Answer from the drawing. Dimensions are ordinates in mm from the lowest x, y and z of the part. Round coordinates to 2 decimals unless told otherwise and drop trailing zeros. Order: outer loops, then holes, each group sorted by start corner. A loop starts at its lowest first (then second) coordinate and runs counter-clockwise, first axis right, second up. Notation, with made-up numbers: (79, 67.25) -> (121, 67.25) arc R14 cw to (121, 74.25) -> close; hole circle Ø5 at (20.25, -2.5). An arc over 180 degrees is marked (long way). Use a Markdown table: item, result. Add a question column.
Item 1: Find the intervals of material crossed by L1, parallel to Z at x = 80, y = 63.5; L2, parallel to Z at x = 46, y = 53, in increasing order. Write a range as [from, to].
Item 2: A flat-ended cylindrical pin translates along its axis: P1, Ø4, axis at x = 98.5, y = 78.5, coming from the -Z side. Find the tip coordinate at first contact, or state that the pin passes through.
Item 3: For a pull along Z with two mould halves and no side action, classify the marked faces 1, 2, 3 and 4 as +Z half, -Z half, draft (parallel to the pull), parting line (faces both ways), or undercut.
Item 4: A cutting plane is placed at A-A, the plane y = 63.5. Determine the outline of the cut face in (x, z), plus the area to 3 significant figures.
Item 5: A cutting plane is placed at C-C, the plane x = 63.5. Determine the outline of the cut face in (y, z).
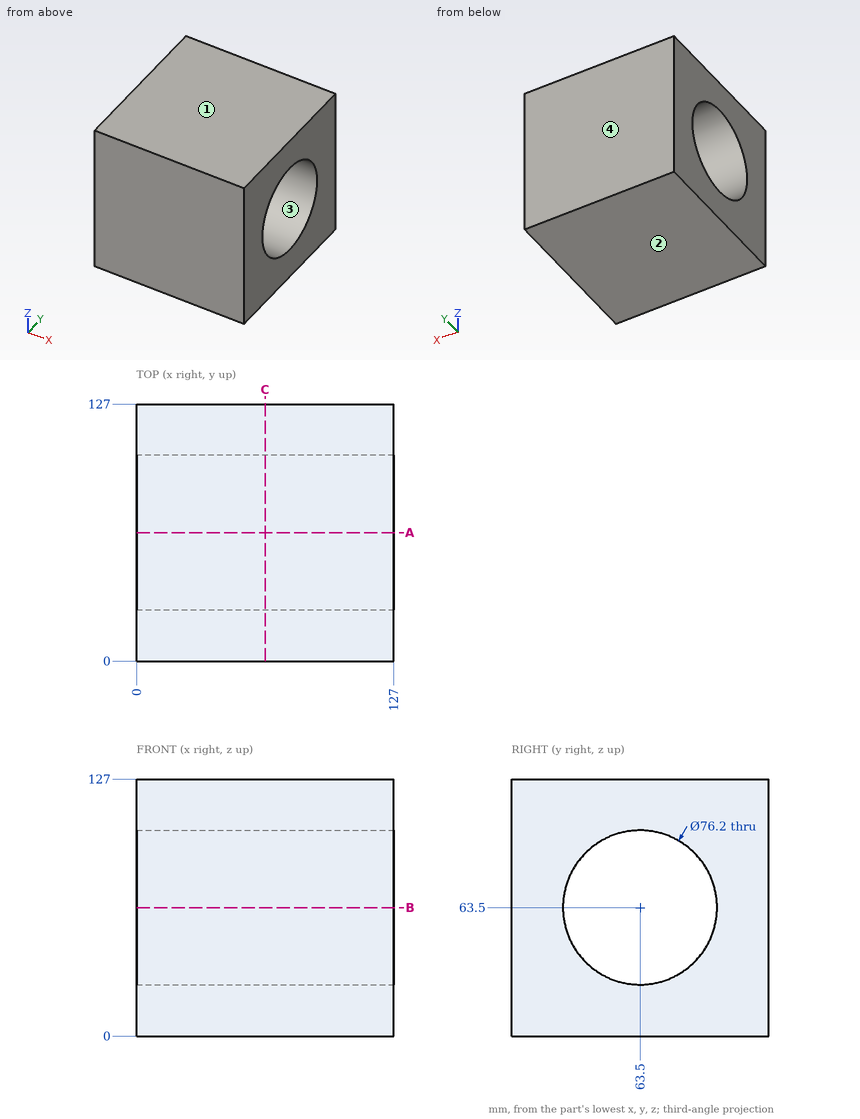
Reported:
| question | item | result |
|---|---|---|
| 1 | L1 | [0, 25.4], [101.6, 127] |
| 1 | L2 | [0, 26.88], [100.12, 127] |
| 2 | P1 | z = 0 |
| 3 | face 1 | +Z half |
| 3 | face 2 | -Z half |
| 3 | face 3 | undercut |
| 3 | face 4 | draft |
| 4 | outline | (0, 0) -> (127, 0) -> (127, 25.4) -> (0, 25.4) -> close; (0, 101.6) -> (127, 101.6) -> (127, 127) -> (0, 127) -> close |
| 4 | area | 6,450 mm² |
| 5 | outline | (0, 0) -> (127, 0) -> (127, 127) -> (0, 127) -> close; hole circle Ø76.2 at (63.5, 63.5) |
